Source: CAD feature listing. Evaluate the final solid. Frame: model axes, mm. A direction names the side the tool comes from. Coordinates: 2 decimals unless noted, no trailing zeros. Write each loop counter-clockwise with the first axis right and the second up, starting at its lowest first coordinate (ties: lowest second). Pieces come first, ordered by that corner, then holes. Notation, with made-up numbers: M -39.5,-36.5 L -9.5,-36.5 A27 ccw -9.5,-19.5 Z; hole C -38.75,3.25 d11. An arc over 180 degrees is marked long. Answer as CSV lines item,"result". Start each with the question number.
1. Section A-A on z = -7.75. Return the cut outline in (x, y).
2. Line query: probe 1 along X at (y, z) = (0.35, -8); probe 2 along Z at (x, y) = (1.5, 1.55); probe 3 along Z at (x, y) = (8.75, 0.35). Output: solid intervals per line, ascending. Write a range as [from, to].
3. Section D-D on x = 2.25. Return the cut outline in (y, z), plus the area to 3 significant figures.
4. Section C-C on y = 2.4. Return the cut outline in (x, z).
5. Mould query, pull axis X, two halves, no side actions, for faces 1 (the face through (0, 1, -10)), 2 (the face through (7.535, 1.521, 4.93)), 3 (the face through (7.5, 1, -8)). Classes: pulls with the +X half, pulls with the -X half, needs draft (parallel to the pull), parting line crosses it, or undercut.
6. Reachability of faces 4 (the face through (-5, 1, -7)), 5 (the face through (2.535, 1.521, 5.07)), 6 (the face through (10, 1, -5)) from +Z, -Z, +X, -X, +Y, -Y: full face, straight path, thin tool, end or side. Return the list, or none.
7. Section B-B on z = 3. Return the cut outline in (x, y).
8. Contact query for flat-ended pins moving along their axis: pin 1 Ø4 at (x, z) = (8, 2) entering from -Y; pin 2 Ø1.5 at (x, y) = (5, 1) entering from -Z. Output: stop coordinate, or through.
```python
from build123d import *

# Parameters (mm, degrees)
SKETCH1_W               = 20
SKETCH1_H               = 20
BOSS_EXTRUDE1_DEPTH     = 3
CUT_EXTRUDE1_DEPTH      = 1
CUT_EXTRUDE1_DEPTH_BACK = 4
CUT_EXTRUDE2_START      = -4
SKETCH3_W               = 5
SKETCH3_H               = 3
CUT_EXTRUDE2_DEPTH      = 5


with BuildPart() as part:
    # Sketch1 → Boss-Extrude1 (new body)
    with BuildSketch(Plane(origin=(0, 0, 0), x_dir=(1, 0, 0), z_dir=(0, 1, 0))):
        Rectangle(SKETCH1_W, SKETCH1_H)
    extrude(amount=BOSS_EXTRUDE1_DEPTH)

    # Sketch2 → Cut-Extrude1 (cut, two sides)
    with BuildSketch(Plane(origin=(0, 3, 0), x_dir=(1, 0, 0), z_dir=(0, 1, 0))) as cut_extrude1_sk:
        Polygon((-5, -10), (-10, 0), (-10, -10), align=None)
        Polygon((0, 0), (-5, -10), (5, -10), align=None)
        Polygon((10, 0), (5, -10), (10, -10), align=None)
    extrude(amount=CUT_EXTRUDE1_DEPTH, mode=Mode.SUBTRACT)
    extrude(cut_extrude1_sk.sketch, amount=-CUT_EXTRUDE1_DEPTH_BACK, mode=Mode.SUBTRACT)

    # Sketch3 → Cut-Extrude2 (cut)
    with BuildSketch(Plane(origin=(0, 3, 0), x_dir=(1, 0, 0), z_dir=(0, 1, 0)).offset(CUT_EXTRUDE2_START)):
        with Locations((-5, 8.5)):
            Rectangle(SKETCH3_W, SKETCH3_H)
    cut_extrude2 = extrude(amount=CUT_EXTRUDE2_DEPTH, mode=Mode.SUBTRACT)

    # Mirror1: Cut-Extrude2 across plane
    add(cut_extrude2.mirror(Plane(origin=(0, 0, 0), x_dir=(0, 0, 1), z_dir=(1, 0, 0))), mode=Mode.SUBTRACT)


solid = part.part
```
Values:
1,outline,"M -10,0 L -7.5,0 L -7.5,3 L -10,3 Z; M -2.5,0 L 2.5,0 L 2.5,3 L -2.5,3 Z; M 7.5,0 L 10,0 L 10,3 L 7.5,3 Z"
2,probe 1,"[-10, -7.5], [-2.5, 2.5], [7.5, 10]"
2,probe 2,"[-10, 3]"
2,probe 3,"[-10, 2.5]"
3,outline,"M 0,-10 L 3,-10 L 3,4.5 L 0,4.5 Z"
3,area,"43.5 mm²"
4,outline,"M -10,-10 L -7.5,-10 L -7.5,-7 L -2.5,-7 L -2.5,-10 L 2.5,-10 L 2.5,-7 L 7.5,-7 L 7.5,-10 L 10,-10 L 10,0 L 5,10 L 0,0 L -5,10 L -10,0 Z"
5,face 1,"needs draft"
5,face 2,"pulls with the +X half"
5,face 3,"undercut"
6,face 4,"-Z, +Y, -Y"
6,face 5,"+Z, +Y, -Y"
6,face 6,"+Z, -Z, +X, +Y, -Y"
7,outline,"M -8.5,0 L -1.5,0 L -1.5,3 L -8.5,3 Z; M 1.5,0 L 8.5,0 L 8.5,3 L 1.5,3 Z"
8,pin 1,"y = 0"
8,pin 2,"z = -7"
